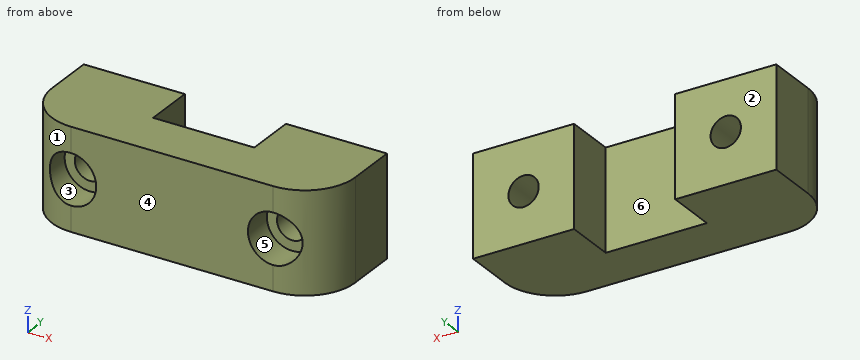
from build123d import *

# Parameters (mm, degrees)
F0_W     = 30
F0_H     = 10
F1_DEPTH = 10
F2_W     = 5
F2_H     = 5
F3_DEPTH = 25
F4_R     = 5
F5_R     = 1.5
F6_DEPTH = 25
F7_R     = 2.5
F8_DEPTH = 3


with BuildPart() as f1:
    # F0 (on Front) → F1 (new body)
    with BuildSketch(Plane.XZ):
        with Locations((-14.225836, 5)):
            Rectangle(F0_W, F0_H)
    extrude(amount=F1_DEPTH)

    # F2 (on face) → F3 (cut)
    with BuildSketch(Plane.XY.offset(10)):
        with Locations((-11.725836, -2.5)):
            Rectangle(F2_W, F2_H)
        with Locations((-16.725836, -2.5)):
            Rectangle(F2_W, F2_H)
    extrude(amount=-F3_DEPTH, mode=Mode.SUBTRACT)

    # F4
    f4_edges = [f1.edges().sort_by_distance(p)[0] for p in [
        (-29.225836, -10, 5),
        (0.774164, -10, 5),
    ]]
    fillet(f4_edges, radius=F4_R)

    # F5 (on face) → F6 (cut)
    with BuildSketch(Plane.XZ.offset(10)):
        with Locations((-24.225836, 5)):
            Circle(F5_R)
        with Locations((-4.225836, 5)):
            Circle(F5_R)
    extrude(amount=-F6_DEPTH, mode=Mode.SUBTRACT)

    # F7 (on face) → F8 (cut)
    with BuildSketch(Plane.XZ.offset(10)):
        with Locations((-24.225836, 5)):
            Circle(F7_R)
        with Locations((-4.225836, 5)):
            Circle(F7_R)
    extrude(amount=-F8_DEPTH, mode=Mode.SUBTRACT)


solid = f1.part
Design review of the part built by this model. Coordinates are the model's own, in mm. Face numbers are marked on the shaded views. A direction names the side the tool comes from. Round coordinates to 2 decimals unless told otherwise and drop trailing zeros. Write each loop counter-clockwise with the first axis right and the second up, starting at its lowest first coordinate (ties: lowest second). Pieces come first, ordered by that corner, then holes.
Item 1: Consider section C-C on x = -3. Give the boundary of the cut face in (y, z).
Item 2: For the marked faces 4, 5 and 6, list the 3-axis set-ups (+Z, -Z, +X, -X, +Y, -Y) from which the entire face can be reached by the end or side of a thin tool; tool diameter is ignored.
Item 3: Consider section B-B on z = 5. Give the boundary of the cut face in (x, y), and give its area (3 significant figures).
Item 4: Consider section D-D on z = 8.75. Give the boundary of the cut face in (x, y), and give its area (3 significant figures).
Item 5: Consider section A-A on y = -3.5. Give the boundary of the cut face in (x, z).
Item 6: For pin 1 Ø4 at (x, z) = (-3.5, 4.5) entering from -Y; pin 2 Ø5 at (y, z) = (-8, 4) entering from -X; pin 3 Ø1 at (x, z) = (-18, 7.5) entering from +Y, all flat-tipped, find the tip position at first contact; note any pin that passes through.
Item 7: Draft analysis for pull direction X (two halves, no side actions). For the marked faces 1, 2 and 3, state which applies: released by +X, released by -X, zero draft, split by the parting line, or undercut.
Item 8: Wall thickness on L1, parallel to X at y = -3.75, z = 6; L2, parallel to X at y = -8.6, z = 5; L3, parallel to X at y = -8.25, z = 5: over which ranges is each line inside the solid? List them lowest first.
Check values:
1. outline: (-9.85, 0) - (0, 0) - (0, 4.14) - (-7, 4.14) - (-7, 2.82) - (-9.85, 2.82) - close; (-9.85, 7.18) - (-7, 7.18) - (-7, 5.86) - (0, 5.86) - (0, 10) - (-9.85, 10) - close
2. face 4: +Z, -Z, +X, -X, -Y
2. face 5: -Y
2. face 6: +Z, -Z, +Y
3. outline: (-29.23, -5) arc R5 ccw to (-26.73, -9.33) - (-26.73, -7) - (-25.73, -7) - (-25.73, 0) - (-29.23, 0) - close; (-22.73, -7) - (-21.73, -7) - (-21.73, -10) - (-6.73, -10) - (-6.73, -7) - (-5.73, -7) - (-5.73, 0) - (-9.23, 0) - (-9.23, -5) - (-19.23, -5) - (-19.23, 0) - (-22.73, 0) - close; (-2.73, -7) - (-1.73, -7) - (-1.73, -9.33) arc R5 ccw to (0.77, -5) - (0.77, 0) - (-2.73, 0) - close
3. area: 168 mm2
4. outline: (-29.23, -5) arc R5 ccw to (-24.23, -10) - (-4.23, -10) arc R5 ccw to (0.77, -5) - (0.77, 0) - (-9.23, 0) - (-9.23, -5) - (-19.23, -5) - (-19.23, 0) - (-29.23, 0) - close
4. area: 239 mm2
5. outline: (-29.23, 0) - (-19.23, 0) - (-19.23, 10) - (-29.23, 10) - close; (-9.23, 0) - (0.77, 0) - (0.77, 10) - (-9.23, 10) - close; hole circle Ø3 at (-24.23, 5); hole circle Ø3 at (-4.23, 5)
6. pin 1: stops at y = -9.99
6. pin 2: stops at x = -29.2
6. pin 3: stops at y = -5
7. face 1: released by -X
7. face 2: zero draft
7. face 3: undercut
8. L1: x = -29.23 to -25.34, -23.11 to -19.23, -9.23 to -5.34, -3.11 to 0.77
8. L2: x = -27.7 to -26.73, -21.73 to -6.73, -1.73 to -0.76
8. L3: x = -28.03 to -26.73, -21.73 to -6.73, -1.73 to -0.43
